from build123d import *

# Parameters (mm, degrees)
F0_W      = 25.4
F0_H      = 25.4
F1_DEPTH  = 38.1
F2_R      = 5.08
F3_R      = 5.08
F1_FACE_W = 15.24
F1_FACE_H = 15.24
F4_DEPTH  = 15.24


with BuildPart() as f1:
    # F0 (on Top) → F1 (new body)
    with BuildSketch(Plane.XY):
        Rectangle(F0_W, F0_H)
    extrude(amount=-F1_DEPTH)

    # F2
    f2_edges = [f1.edges().sort_by_distance(p)[0] for p in [
        (-12.7, 0, -38.1),
    ]]
    fillet(f2_edges, radius=F2_R)

    # F3
    f3_edges = [f1.edges().sort_by_distance(p)[0] for p in [
        (2.54, -12.7, -38.1),
        (-7.62, 0, -38.1),
        (12.7, 0, -38.1),
        (2.54, 12.7, -38.1),
        (-12.7, -12.7, -16.51),
        (-11.212102, -12.7, -36.612102),
        (0, -12.7, 0),
        (12.7, -12.7, -19.05),
        (12.7, 12.7, -19.05),
    ]]
    fillet(f3_edges, radius=F3_R)

    # F1_face (on face) → F4 (join)
    with BuildSketch(Plane(origin=(0, 0, -38.1), x_dir=(1, 0, 0), z_dir=(0, 0, -1))):
        Rectangle(F1_FACE_W, F1_FACE_H)
    extrude(amount=F4_DEPTH)


solid = f1.part
Build history of the part. All positions in model axes, mm. A direction names the side the tool comes from. Round coordinates to 2 decimals unless told otherwise and drop trailing zeros. Write each loop counter-clockwise with the first axis right and the second up, starting at its lowest first coordinate (ties: lowest second). Pieces come first, ordered by that corner, then holes. Notation, with made-up numbers: M 79,53.25 L 88,53.25 A21 ccw 88,89.25 Z; hole C 8,-17.75 d1. An arc over 180 degrees is marked long. Use CSV: the item, a comma, the result in double quotes.
1. Saw through at A-A (x = 3.25). Give the cut face in (y, z).
Reply:
outline,"M -12.7,-33.02 A5.08 ccw -7.62,-38.1 L -7.62,-53.34 L 7.62,-53.34 L 7.62,-38.1 A5.08 ccw 12.7,-33.02 L 12.7,0 L -7.62,0 A5.08 ccw -12.7,-5.08 Z"
2. Saw through at D-D (x = 11.25). Give the cut face in (y, z), plus the area to 3 significant figures.
Reply:
outline,"M -11.17,-33.02 A3.55 ccw -7.62,-36.57 L 7.62,-36.57 A3.55 ccw 11.17,-33.02 L 11.17,0 L -7.62,0 A5.08 ccw -11.17,-1.45 Z"
area,"810 mm²"
3. Flat gauge pins, fed straight in: pin 1 (3 mm diameter, centred on y = 5.5, z = -38.5, fed in from -X); pin 2 (3 mm diameter, centred on x = 6, z = -42, fed in from +Y); pin 3 (4.5 mm diameter, centred on y = 0, z = -49, fed in from -X). Where does each tip first touch, or does it go through?
Reply:
pin 1,"stops at x = -10.78"
pin 2,"stops at y = 7.62"
pin 3,"stops at x = -7.62"
4. Saw through at C-C (y = -2.5). Give the cut face in (x, z), plus the area to 3 significant figures.
Reply:
outline,"M -12.7,-33.02 A5.08 ccw -7.62,-38.1 L -7.62,-53.34 L 7.62,-53.34 L 7.62,-38.1 A5.08 ccw 12.7,-33.02 L 12.7,0 L -12.7,0 Z"
area,"1,190 mm²"
5. Two-plate mould, pull along X, no slides. Class faces 4 (the face through (-7.62, 0, -46)), 5 (the face through (7.62, 0, -46)), 6 (the face through (0, 0, -53.34)): +X half, -X half, draft (parallel to the pull), parting line (faces both ways), or undercut.
Reply:
face 4,"-X half"
face 5,"+X half"
face 6,"draft"
6. Saw through at B-B (z = -9.5). Give the cut face in (x, y).
Reply:
outline,"M -12.7,-7.62 A5.08 ccw -7.62,-12.7 L 7.62,-12.7 A5.08 ccw 12.7,-7.62 L 12.7,7.62 A5.08 ccw 7.62,12.7 L -7.62,12.7 A5.08 ccw -12.7,7.62 Z"
7. Wall check: probe 1 along Y at (x, z) = (-1.5, -44); probe 2 along Z at (x, y) = (3.75, -10.5). Give the ranges that are in metal, low to high. Write a range as from..to.
Reply:
probe 1,"y = -7.62..7.62"
probe 2,"z = -37.2..-0.9"
8. Tool access for faces 1 (the face through (0.178, -11.251, -1.528)), 2 (the face through (0, 7.62, -46)), 3 (the face through (0, -7.62, -46)): list every direction of +Z, -Z, +X, -X, +Y, -Y with a clear straight run to the whole face (end or side of a thin tool).
Reply:
face 1,"+Z, +X, -X, -Y"
face 2,"-Z, +X, -X, +Y"
face 3,"-Z, +X, -X, -Y"
